Autodesk Inventor part; units mm, degrees
ref_plane "YZ Plane" through (0, 0, 0) normal (1, 0, 0) x (0, 1, 0)
ref_plane "XZ Plane" through (0, 0, 0) normal (0, 1, 0) x (-1, 0, 0)
ref_plane "XY Plane" through (0, 0, 0) normal (0, 0, 1) x (1, 0, 0)
ref_plane "Work Plane1" through (0, 0, 0) normal (0, 0, 1) x (1, 0, 0)
ref_plane "Work Plane2" through (0, 0, 0) normal (0, 0, 1) x (1, 0, 0)
sketch "Sketch6" plane through (0, 0, 0) normal (0, 0, 1) x (1, 0, 0)
  line L0 (20, 33.25) -> (1.5, 33.25)
  line L1 (20, 33.25) -> (20, 108.5)
  line L2 (1.5, 108.5) -> (20, 108.5)
  line L3 (1.5, 33.25) -> (1.5, 44.75)
  circle A0 centre (10.5, 63.5) radius 2.1
  circle A1 centre (10.5, 53.5) radius 2.1
  line L4 (20, 73.5) -> (-19.5, 73.5)
  line L5 (-19.5, 73.5) -> (-19.5, 43.5)
  line L6 (-19.5, 43.5) -> (20, 43.5)
  line L7 (20, 43.5) -> (20, 73.5)
  line L8 (-71.5, 45.5) -> (-71.5, 108.5)
  line L9 (-19.5, 73.5) -> (1.5, 73.5)
  line L10 (1.5, 73.5) -> (1.5, 56.5)
  line L11 (1.5, 56.5) -> (-19.5, 56.5)
  line L12 (-19.5, 56.5) -> (-19.5, 73.5)
  line L13 (-10.5, 43.5) -> (-19.5, 43.5)
  line L14 (-19.5, 43.5) -> (-19.5, 56.5)
  line L15 (-19.5, 56.5) -> (-10.5, 56.5)
  line L16 (-10.5, 56.5) -> (-10.5, 43.5)
  line L17 (4.5, 44.75) -> (1.5, 44.75)
  line L18 (1.5, 56.25) -> (1.5, 108.5)
  line L19 (1.5, 56.25) -> (4.5, 56.25)
  line L20 (4.5, 56.25) -> (4.5, 44.75)
  point P0 (0, 0)
  point P1 (20, 43.5)
  point P2 (-71.5, 60.5)
  point P3 (1.5, 73.5)
  point P4 (1.5, 43.5)
  point P5 (1.5, 73.5)
  point P6 (1.5, 73.5)
  dimension "d28" = 10
  dimension "d29" = 10
  dimension "d92" = 30
  dimension "d94" = 17
  dimension "d95" = 9
extrude "Extrusion5" add sketch "Sketch6" along normal blind 7 contours L6 L3 L17 L20 L19 L18 L10 L4 L1 | L6 L16 L11 L18 L19 L20 L17 L3
ref_plane "Work Plane3" through (0, 0, 22) normal (0, 0, 1) x (1, 0, 0)
ref_plane "Work Plane4" through (0, 0, 17) normal (0, 0, 1) x (1, 0, 0)
sketch "Sketch17" plane through (0, 0, 17) normal (0, 0, 1) x (1, 0, 0)
  line L0 (-13, 58.5) -> (0, 58.5)
  line L1 (0, 58.5) -> (0, 88.5)
  line L2 (0, 88.5) -> (-13, 88.5)
  line L3 (-13, 88.5) -> (-13, 58.5)
  circle A0 centre (-5.7, 50.5) radius 2.8
  line L4 (1.5, 56.5) -> (-10.5, 56.5)
  line L5 (20, 43.5) -> (20, 73.5)
  line L6 (20, 73.5) -> (1.5, 73.5)
  line L7 (-10.5, 43.5) -> (20, 43.5)
  line L8 (-10.5, 56.5) -> (-10.5, 43.5)
  line L9 (1.5, 73.5) -> (1.5, 56.5)
  line L10 (1.5, 56.5) -> (-10.5, 56.5)
  point P0 (0, 0)
  point P1 (-6.5, 58.5)
  dimension "d75" = 7.3
  dimension "d88" = 5.6
  dimension "d103" = 7
extrude "Extrusion16" cut sketch "Sketch17" against normal through all contours A0
fillet "Fillet8" radius 4 3 edges at (20, 73.5, 3.5) (20, 43.5, 3.5) (1.5, 73.5, 3.5)
sketch "Sketch19" plane through (0, 0, 7) normal (0, 0, 1) x (1, 0, 0)
  line L0 (20, 47.5) -> (20, 69.5)
  line L1 (16, 73.5) -> (5.5, 73.5)
  line L2 (-10.5, 43.5) -> (16, 43.5)
  line L3 (-10.5, 43.5) -> (16, 43.5)
  line L4 (-10.5, 56.5) -> (1.5, 56.5)
  line L5 (1.5, 56.5) -> (1.5, 43.5)
  line L6 (1.5, 43.5) -> (-10.5, 43.5)
  line L7 (-10.5, 43.5) -> (-10.5, 56.5)
  circle A0 centre (-5.7, 50.5) radius 2.8
  arc A1 (16, 43.5) -> (20, 47.5) centre (16, 47.5) ccw
  arc A2 (20, 69.5) -> (16, 73.5) centre (16, 69.5) ccw
  line L8 (1.5, 69.5) -> (1.5, 56.5)
  line L9 (1.5, 56.5) -> (-10.5, 56.5)
  line L10 (-10.5, 56.5) -> (-10.5, 43.5)
  arc A3 (5.5, 73.5) -> (1.5, 69.5) centre (5.5, 69.5) ccw
  point P0 (0, 0)
  point P1 (1.5, 43.5)
  point P2 (-15.5, 43.5)
  dimension "d99" = 18.5
extrude "Extrusion18" add sketch "Sketch19" along normal blind 3 contours L2 L7 L4 L5
fillet "Fillet10" radius 2 4 edges at (-10.5, 56.5, 5) (1.5, 43.5, 8.5) (-10.5, 43.5, 5) (1.5, 56.5, 3.5)
properties part number "base-tensioner_3DPrint"
Source: CAD feature listing. Evaluate the final solid. Frame: model axes, mm. A direction names the side the tool comes from. Give positions to 0.01 mm unless a question says otherwise; leave off trailing zeros. Order: outer loops, then holes, each group sorted by start corner. A loop starts at its lowest first (then second) coordinate and runs counter-clockwise, first axis right, second up. Notation, with made-up numbers: (2, 62.25) -> (48, 62.25) arc R20 cw to (48, 70.25) -> close; hole circle Ø4 at (-39, 64). An arc over 180 degrees is marked (long way). Use a Markdown table: item, result.
Q1. Section C-C (z = 5). Return the cut outline in (x, y).
A:
| item | result |
|---|---|
| outline | (-10.5, 45.5) arc R2 ccw to (-8.5, 43.5) -> (16, 43.5) arc R4 ccw to (20, 47.5) -> (20, 69.5) arc R4 ccw to (16, 73.5) -> (5.5, 73.5) arc R4 ccw to (1.5, 69.5) -> (1.5, 58.5) arc R2 cw to (-0.5, 56.5) -> (-8.5, 56.5) arc R2 ccw to (-10.5, 54.5) -> close; hole circle Ø5.6 at (-5.7, 50.5); hole circle Ø4.2 at (10.5, 53.5); hole circle Ø4.2 at (10.5, 63.5) |
Q2. Pull-direction query (Y, two-part tool) for faces 4 (the face through (0.9, 57.07, 3.55)), 5 (the face through (12, 59, 7)), 6 (the face through (-6.307, 53.233, 4.93)); classes: +Y half, -Y half, draft (parallel to the pull), parting line (faces both ways), or undercut.
A:
| item | result |
|---|---|
| face 4 | +Y half |
| face 5 | draft |
| face 6 | undercut |
Q3. Section B-B (y = 63.5). Return the cut outline in (x, z).
A:
| item | result |
|---|---|
| outline | (1.5, 0) -> (8.4, 0) -> (8.4, 7) -> (1.5, 7) -> close; (12.6, 0) -> (20, 0) -> (20, 7) -> (12.6, 7) -> close |
Q4. Material intervals for line 1 (Y direction, x = 10.5, z = 4); line 2 (Y direction, x = -5.7, z = 5.5); line 3 (Y direction, x = -1, z = 1.25), sorted ascending. Write a range as [from, to].
A:
| item | result |
|---|---|
| line 1 | [43.5, 51.4], [55.6, 61.4], [65.6, 73.5] |
| line 2 | [43.5, 47.7], [53.3, 56.5] |
| line 3 | [43.5, 56.5] |
Q5. Section D-D (x = 10.5). Return the cut outline in (y, z), and give its area (3 significant figures).
A:
| item | result |
|---|---|
| outline | (43.5, 0) -> (51.4, 0) -> (51.4, 7) -> (43.5, 7) -> close; (55.6, 0) -> (61.4, 0) -> (61.4, 7) -> (55.6, 7) -> close; (65.6, 0) -> (73.5, 0) -> (73.5, 7) -> (65.6, 7) -> close |
| area | 151 mm^2 |
Q6. Access query for faces 1 (the face through (1.5, 64, 3)), 2 (the face through (0.9, 44.07, 8.52)), 3 (the face through (20, 58, 3)). Directions: +Z, -Z, +X, -X, +Y, -Y. A direction counts if a zero-diameter tool reaches every point of the face in a straight line with its end or side. Return the directions, or none.
A:
| item | result |
|---|---|
| face 1 | +Z, -Z, -X, +Y |
| face 2 | +Z, +X, -Y |
| face 3 | +Z, -Z, +X, +Y, -Y |
Q7. First-contact query: P1, Ø4, axis at y = 62.5, z = 6, coming from the -X side; P2, Ø1, axis at x = 16, y = 57, coming from the +Z side. Flat tips, straight axial feed; report the tip coordinate or a pass-through.
A:
| item | result |
|---|---|
| P1 | x = 1.5 |
| P2 | z = 7 |
Q8. Section A-A (x = -5.7). Return the cut outline in (y, z), and give its area (3 significant figures).
A:
| item | result |
|---|---|
| outline | (43.5, 0) -> (47.7, 0) -> (47.7, 10) -> (43.5, 10) -> close; (53.3, 0) -> (56.5, 0) -> (56.5, 10) -> (53.3, 10) -> close |
| area | 74.0 mm^2 |
